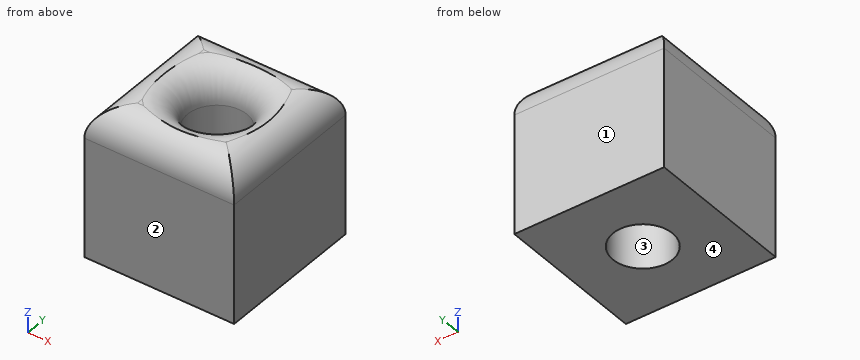
from build123d import *

# Parameters (mm, degrees)
F0_W        = 25
F0_H        = 25
F1_DEPTH    = 25
F2_R        = 4.9593089968
F3_DEPTH    = 25.4
F4_T1_DEPTH = 50.4
F4_T3_DEPTH = 50.4


# Not quite as in the source:
# - a fillet or chamfer that OpenCascade refuses, or shapes differently, is made with other operations: its cross-section is extruded or revolved along the edge and cut away or added


with BuildPart() as f1:
    # F0 (on Top) → F1 (new body)
    with BuildSketch(Plane.XY):
        with Locations((-12.5, -12.5)):
            Rectangle(F0_W, F0_H)
    extrude(amount=F1_DEPTH)

    # F2 (on face) → F3 (cut)
    with BuildSketch(Plane.XY.offset(25)):
        with Locations((-12.1455704793, -12.4741084874)):
            Circle(F2_R)
    extrude(amount=-F3_DEPTH, mode=Mode.SUBTRACT)

    # F4: fillet of radius 5.08 on 5 edges, made by hand

    # F4_s2 → F4_t1 (cut)
    with BuildSketch(Plane.XZ.offset(-12.7)):
        with BuildLine():
            ThreePointArc((0, 19.92), (-1.4878975516, 23.5121024484), (-5.08, 25))
            Line((-5.08, 25), (0, 25))
            Line((0, 25), (0, 19.92))
        make_face()
        with BuildLine():
            ThreePointArc((-19.92, 25), (-23.5121024484, 23.5121024484), (-25, 19.92))
            Line((-25, 19.92), (-25, 25))
            Line((-25, 25), (-19.92, 25))
        make_face()
    extrude(amount=F4_T1_DEPTH, mode=Mode.SUBTRACT)

    # F4_s4 → F4_t3 (cut)
    with BuildSketch(Plane.YZ.offset(-37.7)):
        with BuildLine():
            ThreePointArc((-25, 19.92), (-23.5121024484, 23.5121024484), (-19.92, 25))
            Line((-19.92, 25), (-25, 25))
            Line((-25, 25), (-25, 19.92))
        make_face()
        with BuildLine():
            ThreePointArc((0, 19.92), (-1.4878975516, 23.5121024484), (-5.08, 25))
            Line((-5.08, 25), (0, 25))
            Line((0, 25), (0, 19.92))
        make_face()
    extrude(amount=F4_T3_DEPTH, mode=Mode.SUBTRACT)

    # F4_s5 → F4_t6 (revolve, cut)
    with BuildSketch(Plane.XZ.offset(12.4741084874)):
        with BuildLine():
            ThreePointArc((-2.1062614826, 25), (-5.698363931, 23.5121024484), (-7.1862614826, 19.92))
            Line((-7.1862614826, 19.92), (-7.1862614826, 25))
            Line((-7.1862614826, 25), (-2.1062614826, 25))
        make_face()
    revolve(axis=Axis((-12.1455704793, -12.4741084874, 25), (0, 0, 1)), mode=Mode.SUBTRACT)


solid = f1.part
For this review, take the finished solid that the model builds, in its own axes (mm). Face numbers are marked on the shaded views. Round coordinates to 2 decimals unless told otherwise and drop trailing zeros. Loops run counter-clockwise (first coordinate to the right, second up) from the corner with the lowest first, then second, coordinate; pieces in that order, holes last. Notation, with made-up numbers: (74, 34) - (133, 34) arc R13 cw to (133, 54) - close; hole circle Ø2 at (-37.5, -23). An arc over 180 degrees is marked (long way). One line per question, with ' | ' between items.
Q1. For line 1 along Y through (x, z) = (-15.5, 1.5); line 2 along X through (y, z) = (-16, 19.75); line 3 along X through (y, z) = (-13, 17), list the stretches that pass through material, from the lowest coordinate up. Write a range as [from, to].
Taken from the geometry:
line 1: y = [-25, -16.13], [-8.82, 0] | line 2: x = [-25, -15.63], [-8.66, 0] | line 3: x = [-25, -17.08], [-7.21, 0]
Q2. Take a section at D-D (z = 17). Give the boundary of the cut face in (x, y), and give its area (3 significant figures).
Taken from the geometry:
outline: (-25, -25) - (0, -25) - (0, 0) - (-25, 0) - close; hole circle Ø9.92 at (-12.15, -12.47) | area: 548 mm²
Q3. The part is to be moulded in two halves that separate along Y. For the marked faces 1, 2, 3 and 4, say which applies: released by +Y, released by -Y, zero draft, split by the parting line, or undercut.
Taken from the geometry:
face 1: released by +Y | face 2: released by -Y | face 3: undercut | face 4: zero draft
Q4. Take a section at B-B (y = -1.75). Give the boundary of the cut face in (x, z).
Taken from the geometry:
outline: (-25, 0) - (0, 0) - (0, 19.92) arc R5.08 ccw to (-1.75, 23.76) - (-23.25, 23.76) arc R5.08 ccw to (-25, 19.92) - close
Q5. Take a section at C-C (x = -22.75). Give the boundary of the cut face in (y, z).
Taken from the geometry:
outline: (-25, 0) - (0, 0) - (0, 19.92) arc R5.08 ccw to (-2.25, 24.14) - (-22.75, 24.14) arc R5.08 ccw to (-25, 19.92) - close
Q6. For pin 1 (5 mm diameter, centred on x = -6.5, y = -15, fed in from +Z); pin 2 (2 mm diameter, centred on x = -15.5, y = -13, fed in from -Z); pin 3 (3 mm diameter, centred on x = -6, y = -14.5, fed in from +Z), all flat-tipped, find the tip position at first contact; note any pin that passes through.
Taken from the geometry:
pin 1: stops at z = 24.82 | pin 2: passes through | pin 3: stops at z = 24.56
Q7. Take a section at A-A (z = 20.75). Give the boundary of the cut face in (x, y).
Taken from the geometry:
outline: (-24.93, -24.93) - (-0.07, -24.93) - (-0.07, -0.07) - (-24.93, -0.07) - close; hole circle Ø10.06 at (-12.15, -12.47)
